```python
from build123d import *
from build123d.topology import SkipClean

# Parameters (mm, degrees)
ESBO_O1_R                = 1.65
RESSALTO_EXTRUS_O1_DEPTH = 3
RESSALTO_EXTRUS_O2_START = 15
ESBO_O2_R                = 1.65
RESSALTO_EXTRUS_O2_DEPTH = 15
CORTE_EXTRUS_O1_DEPTH    = 15
RESSALTO_EXTRUS_O3_DEPTH = 2
ESBO_O6_W                = 23.468316857
ESBO_O6_H                = 21.298976644
CORTE_EXTRUS_O2_DEPTH    = 21
ESBO_O7_W                = 18
ESBO_O7_H                = 18
RESSALTO_EXTRUS_O4_DEPTH = 2
CORTE_EXTRUS_O3_DEPTH    = 5
ESBO_O9_W                = 18
ESBO_O9_H                = 2
CORTE_EXTRUS_O4_DEPTH    = 8
ESBO_O10_W               = 18
ESBO_O10_H               = 4
RESSALTO_EXTRUS_O5_DEPTH = 7.5
ESBO_O11_R               = 1.65
CORTE_EXTRUS_O5_DEPTH    = 7.5
ESBO_O12_W               = 18
ESBO_O12_H               = 4
RESSALTO_EXTRUS_O6_DEPTH = 1.5
FILETE1_R                = 6
ESBO_O13_W               = 18
ESBO_O13_H               = 2.5
CORTE_EXTRUS_O6_DEPTH    = 1
ESBO_O14_W               = 18
ESBO_O14_H               = 9
CORTE_EXTRUS_O7_DEPTH    = 1


with BuildPart() as part:
    # Esboço1 → Ressalto-extrusão1 (new body)
    # profile 1 of 3: a face of its own
    with BuildSketch(Plane.XY):
        Polygon((-7, 15.25), (-9, 15.25), (-9, 13.25), (-9, 5), (-6.541451884, 0), (-2.020725942, -6), (2.020725942, -6), (6.541451884, 0), (9, 5), (9, 15.25), (7, 15.25), align=None)
        Polygon((2.020725942, -3.5), (4.041451884, 0), (2.020725942, 3.5), (-2.020725942, 3.5), (-4.041451884, 0), (-2.020725942, -3.5), align=None, mode=Mode.SUBTRACT)
        Polygon((-7, 13.25), (-7, 5), (0, 5), (7, 5), (7, 13.25), align=None, mode=Mode.SUBTRACT)
    # profile 2 of 3: a face of its own
    with BuildSketch(Plane.XY):
        Polygon((7, 13.25), (-7, 13.25), (-7, 5), (0, 5), (7, 5), align=None)
    # profile 3 of 3: a face of its own
    with BuildSketch(Plane.XY):
        Polygon((-2.020725942, -3.5), (2.020725942, -3.5), (4.041451884, 0), (2.020725942, 3.5), (-2.020725942, 3.5), (-4.041451884, 0), align=None)
        Circle(ESBO_O1_R, mode=Mode.SUBTRACT)
    extrude(amount=RESSALTO_EXTRUS_O1_DEPTH)

    # Esboço2 → Ressalto-extrusão2 (add)
    # profile 1 of 2: a face of its own
    with SkipClean():  # the faces are left unmerged after this step: merging them gives an invalid solid
        with BuildSketch(Plane(origin=(0, 0, 0), x_dir=(-1, 0, 0), z_dir=(0, 0, -1)).offset(RESSALTO_EXTRUS_O2_START)):
            Polygon((9, 5), (9, 15.25), (-9, 15.25), (-9, 5), (-6.541451884, 0), (-2.020725942, -6), (2.020725942, -6), (6.541451884, 0), align=None)
            Polygon((7, 5), (7, 13.25), (-7, 13.25), (-7, 5), (0, 5), align=None, mode=Mode.SUBTRACT)
            Polygon((-4.041451884, 0), (-2.020725942, -3.5), (2.020725942, -3.5), (4.041451884, 0), (2.020725942, 3.5), (-2.020725942, 3.5), align=None, mode=Mode.SUBTRACT)
        # profile 2 of 2: a face of its own
        with BuildSketch(Plane(origin=(0, 0, 0), x_dir=(-1, 0, 0), z_dir=(0, 0, -1)).offset(RESSALTO_EXTRUS_O2_START)):
            Polygon((-2.020725942, 3.5), (-4.041451884, 0), (-2.020725942, -3.5), (2.020725942, -3.5), (4.041451884, 0), (2.020725942, 3.5), align=None)
            Circle(ESBO_O2_R, mode=Mode.SUBTRACT)
        extrude(amount=-RESSALTO_EXTRUS_O2_DEPTH)

    # Esboço3 → Corte-extrusão1 (cut)
    with SkipClean():  # the faces are left unmerged after this step: merging them gives an invalid solid
        with BuildSketch(Plane(origin=(0, 0, -15), x_dir=(-1, 0, 0), z_dir=(0, 0, -1))):
            Polygon((-9, 10.625), (-9, 9.125), (-9, 7.625), (-7, 7.625), (-7, 10.625), align=None)
            Polygon((9, 7.625), (9, 9.125), (9, 10.625), (7, 10.625), (7, 7.625), align=None)
        extrude(amount=-CORTE_EXTRUS_O1_DEPTH, mode=Mode.SUBTRACT)

    # Esboço5 → Ressalto-extrusão3 (add)
    with SkipClean():  # the faces are left unmerged after this step: merging them gives an invalid solid
        with BuildSketch(Plane(origin=(0, 0, 0), x_dir=(-1, 0, 0), z_dir=(0, 0, -1))):
            Polygon((-1.583333333, 13.25), (-2.333333333, 13.25), (-3.083333333, 13.25), (-3.083333333, 5), (-1.583333333, 5), align=None)
        extrude(amount=RESSALTO_EXTRUS_O3_DEPTH)

    # Esboço6 → Corte-extrusão2 (cut)
    with BuildSketch(Plane(origin=(0, -16, 0), x_dir=(-1, 0, 0), z_dir=(0, -1, 0))):
        with Locations((-0.042259875, 5.70418088)):
            Rectangle(ESBO_O6_W, ESBO_O6_H)
    extrude(amount=-CORTE_EXTRUS_O2_DEPTH, mode=Mode.SUBTRACT)

    # Esboço7 → Ressalto-extrusão4 (add)
    with BuildSketch(Plane.XZ.offset(-5)):
        with Locations((0, -6)):
            Rectangle(ESBO_O7_W, ESBO_O7_H)
    extrude(amount=RESSALTO_EXTRUS_O4_DEPTH)

    # Esboço8 → Corte-extrusão3 (cut)
    with BuildSketch(Plane(origin=(0, 0, -15), x_dir=(-1, 0, 0), z_dir=(0, 0, -1))):
        Polygon((7, 7.625), (7, 5), (-7, 5), (-7, 7.625), (-9, 7.625), (-9, 3), (9, 3), (9, 7.625), align=None)
        Polygon((7, 10.625), (9, 10.625), (9, 15.25), (-9, 15.25), (-9, 10.625), (-7, 10.625), (-7, 13.25), (7, 13.25), align=None)
    extrude(amount=-CORTE_EXTRUS_O3_DEPTH, mode=Mode.SUBTRACT)

    # Esboço9 → Corte-extrusão4 (cut)
    with BuildSketch(Plane(origin=(0, 0, -10), x_dir=(-1, 0, 0), z_dir=(0, 0, -1))):
        with Locations((0, 14.25)):
            Rectangle(ESBO_O9_W, ESBO_O9_H)
    extrude(amount=-CORTE_EXTRUS_O4_DEPTH, mode=Mode.SUBTRACT)

    # Esboço10 → Ressalto-extrusão5 (add)
    with BuildSketch(Plane.XZ.offset(-3)):
        with Locations((0, 1)):
            Rectangle(ESBO_O10_W, ESBO_O10_H)
    extrude(amount=RESSALTO_EXTRUS_O5_DEPTH)

    # Esboço11 → Corte-extrusão5 (cut)
    with BuildSketch(Plane(origin=(0, 0, -1), x_dir=(-1, 0, 0), z_dir=(0, 0, -1))):
        with Locations((0, -2.8)):
            Circle(ESBO_O11_R)
    extrude(amount=-CORTE_EXTRUS_O5_DEPTH, mode=Mode.SUBTRACT)

    # Esboço12 → Ressalto-extrusão6 (add)
    with BuildSketch(Plane.XZ.offset(4.5)):
        with Locations((0, 1)):
            Rectangle(ESBO_O12_W, ESBO_O12_H)
    extrude(amount=RESSALTO_EXTRUS_O6_DEPTH)

    # Filete1
    filete1_edges = [part.edges().sort_by_distance(p)[0] for p in [
        (-9, -6, 1),
        (9, -6, 1),
    ]]
    fillet(filete1_edges, radius=FILETE1_R)

    # Esboço13 → Corte-extrusão6 (cut)
    with BuildSketch(Plane(origin=(0, 13.25, 0), x_dir=(1, 0, 0), z_dir=(0, 1, 0))):
        with Locations((0, 3.25)):
            Rectangle(ESBO_O13_W, ESBO_O13_H)
    extrude(amount=-CORTE_EXTRUS_O6_DEPTH, mode=Mode.SUBTRACT)

    # Esboço14 → Corte-extrusão7 (cut)
    with BuildSketch(Plane.XZ.offset(-3)):
        with Locations((0, -5.5)):
            Rectangle(ESBO_O14_W, ESBO_O14_H)
    extrude(amount=-CORTE_EXTRUS_O7_DEPTH, mode=Mode.SUBTRACT)


solid = part.part
```
Input: part model. Units: mm. Frame: model coordinates. A direction names the side the tool comes from. Round coordinates to 2 decimals unless told otherwise and drop trailing zeros. Write each loop counter-clockwise with the first axis right and the second up, starting at its lowest first coordinate (ties: lowest second). Pieces come first, ordered by that corner, then holes. Notation, with made-up numbers: (10, -8) - (65, -8) arc R12 cw to (65, -3) - close; hole circle Ø2 at (-37, 39). An arc over 180 degrees is marked (long way). Write item = value, one per line.
(1) Pull-direction query (X, two-part tool) for faces 6 (the flat face through (-9, 6, -2)), 7 (the flat face through (0, 5, 3)), 8 (the flat face through (-3, 13.25, -1)); classes: +X half, -X half, draft (parallel to the pull), parting line (faces both ways), or undercut.
Geometry check:
face_6 = -X half
face_7 = draft
face_8 = undercut
(2) Contact query for flat-ended pins moving along their axis: pin 1 Ø4 at (x, z) = (1.5, -6) entering from -Y; pin 2 Ø1 at (x, z) = (5.5, -1) entering from -Y; pin 3 Ø0.6 at (x, z) = (7.5, -2.5) entering from +Y. Output: stop coordinate, or through.
Geometry check:
pin_1 = 4
pin_2 = -5.66
pin_3 = 12.25
(3) Material intervals for probe 1 along Y at (x, z) = (0, -0.2); probe 2 along Y at (x, z) = (0, 1.85); probe 3 along Y at (x, z) = (0, -1.75), sorted ascending.
Geometry check:
probe_1 = -6 to -4.45, -1.15 to 5, 13.25 to 15.25
probe_2 = -6 to -4.45, -1.15 to 15.25
probe_3 = 4 to 5, 13.25 to 15.25
(4) Section query C-C on y = -2.8. Output: boundary loops of the cut face in (x, z), then the cut area to 3 significant figures.
Geometry check:
outline = (-8.31, -1) - (-1.65, -1) - (-1.65, 3) - (-8.31, 3) - close; (1.65, -1) - (8.31, -1) - (8.31, 3) - (1.65, 3) - close
area = 53.3 mm^2
(5) Access query for faces 1 (the flat face through (8, 13.25, -7)), 2 (the flat face through (-0.1, -0.9, -1)), 3 (the flat face through (-8, 7.625, -5)), 4 (the flat face through (8, 7.625, -5)), 5 (the flat face through (3.083, 9, -1)). Directions: +Z, -Z, +X, -X, +Y, -Y. A direction counts if a zero-diameter tool reaches every point of the face in a straight line with its end or side. Return the directions, or none.
Geometry check:
face_1 = -Z, +X, -X, +Y
face_2 = -Z, +X, -X, -Y
face_3 = -Z, -X
face_4 = -Z, +X
face_5 = -Z
(6) Section query D-D on y = 6. Output: boundary loops of the cut face in (x, z), then the cut area to 3 significant figures.
Geometry check:
outline = (-9, -10) - (-7, -10) - (-7, 0) - (1.58, 0) - (1.58, -2) - (3.08, -2) - (3.08, 0) - (7, 0) - (7, -10) - (9, -10) - (9, 3) - (-9, 3) - close
area = 97.0 mm^2
(7) Section query A-A on z = -6.25. Output: boundary loops of the cut face in (x, y) (3 decimals), then the cut area to 3 significant figures.
Geometry check:
outline = (-9, 4) - (9, 4) - (9, 7.625) - (7, 7.625) - (7, 5) - (-7, 5) - (-7, 7.625) - (-9, 7.625) - close; (-9, 10.625) - (-7, 10.625) - (-7, 13.25) - (-9, 13.25) - close; (7, 10.625) - (9, 10.625) - (9, 13.25) - (7, 13.25) - close
area = 39.0 mm^2
(8) Section query B-B on x = 0. Output: boundary loops of the cut face in (y, z).
Geometry check:
outline = (-6, -1) - (-4.45, -1) - (-4.45, 3) - (-6, 3) - close; (-1.15, -1) - (4, -1) - (4, -10) - (5, -10) - (5, 0) - (13.25, 0) - (13.25, -2) - (15.25, -2) - (15.25, 3) - (-1.15, 3) - close
